The figure shows three views and two pictorial views of one solid part (mm, origin at its lowest corner). Answer the questions. A direction names the side the tool comes from. Coordinates: 2 decimals unless noted, no trailing zeros. Order: outer loops, then holes, each group sorted by start corner. A loop starts at its lowest first (then second) coordinate and runs counter-clockwise, first axis right, second up.
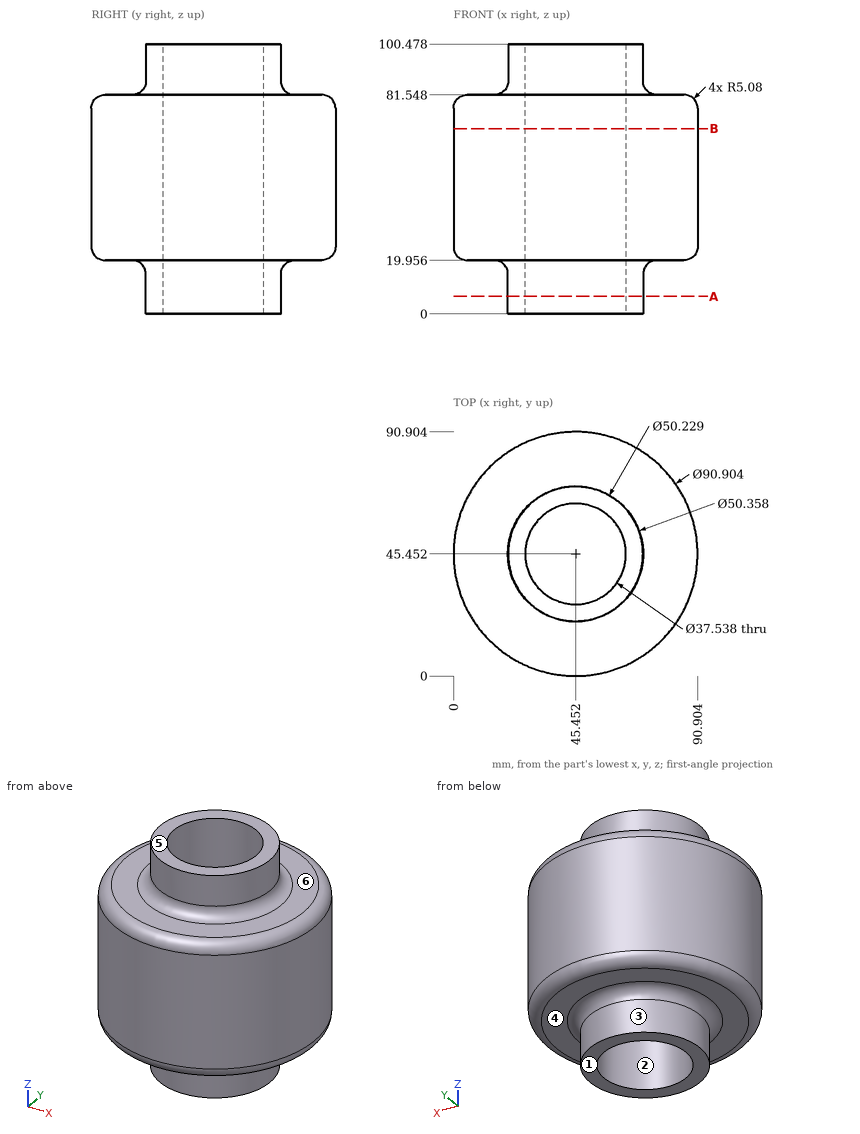
1) Straight lines are drawn through the part: probe 1 along Z at (x, y) = (69, 19.5); probe 2 along Y at (x, z) = (62, 68) (1 decimal); probe 3 along Y at (x, z) = (52.5, 96.5). For each, find the intervals that lie inside material, in ascending order.
2) A cutting plane is placed at B-B, the plane z = 69. Write down the section's boundary in (x, y) (1 decimal).
3) For the marked faces 4, 5 and 6, determine the directions among +Z, -Z, +X, -X, +Y, -Y from which every point of the face is accessible in a straight line to the end or side of a thin tool.
4) A cutting plane is placed at A-A, the plane z = 6.5. Write down the section's boundary in (x, y), plus the area to 3 significant figures.
5) Each of these flat-tipped pins is pushed along its axis until it touches: P1, Ø4, axis at y = 55.5, z = 41, coming from the +X side; P2, Ø2, axis at y = 9.5, z = 64, coming from the +X side; P3, Ø12, axis at y = 18.5, z = 84, coming from the -X side (1 decimal). Where does it stop, or does it pass through?
6) The mould has two halves that part along X. Classify the marked faces 1, 2 and 3: released by +X, released by -X, zero draft, split by the parting line, or undercut.
Working result:
1. probe 1: z = 19.96 to 81.55
1. probe 2: y = 3.1 to 36.6, 54.3 to 87.8
1. probe 3: y = 21.35 to 28.06, 62.85 to 69.56
2. outline: circle Ø90.9 at (45.5, 45.5); hole circle Ø37.5 at (45.5, 45.5)
3. face 4: -Z
3. face 5: +Z, +X, -X, +Y, -Y
3. face 6: +Z
4. outline: circle Ø50.36 at (45.45, 45.45); hole circle Ø37.54 at (45.45, 45.45)
4. area: 885 mm2
5. P1: stops at x = 90.19
5. P2: stops at x = 74.51
5. P3: stops at x = 7.4
6. face 1: zero draft
6. face 2: undercut
6. face 3: split by the parting line
